Design review of the part built by this model. Coordinates are the model's own, in mm. A direction names the side the tool comes from. Give positions to 0.01 mm unless a question says otherwise; leave off trailing zeros. Loops run counter-clockwise (first coordinate to the right, second up) from the corner with the lowest first, then second, coordinate; pieces in that order, holes last.
from build123d import *

# Parameters (mm, degrees)
F0_R     = 2.38125
F0_W     = 0.79375
F0_H     = 1.5875
F1_DEPTH = 3.175
F2_DEPTH = 4.7625


with BuildPart() as f1:
    # F0 (on Top) → F1 (new body)
    with BuildSketch(Plane.XY):
        Polygon((3.96875, 3.96875), (-3.96875, 3.96875), (-3.96875, -3.96875), (-1.5875, -3.96875), (-0.79375, -3.96875), (0, -3.96875), (0.79375, -3.96875), (1.5875, -3.96875), (3.96875, -3.96875), align=None)
        Circle(F0_R, mode=Mode.SUBTRACT)
        Polygon((-0.79375, -3.96875), (-1.5875, -3.96875), (-1.5875, -5.55625), (0, -5.55625), (0, -3.96875), align=None)
        Polygon((1.5875, -5.55625), (1.5875, -3.96875), (0.79375, -3.96875), (0, -3.96875), (0, -5.55625), align=None)
        with BuildLine():
            Line((1.5875, -6.162621), (1.5875, -5.55625))
            Line((1.5875, -5.55625), (0, -5.55625))
            ThreePointArc((0, -5.55625), (0.849683, -5.713002), (1.5875, -6.162621))
        make_face()
        with BuildLine():
            Line((0, -5.55625), (-1.5875, -5.55625))
            Line((-1.5875, -5.55625), (-1.5875, -6.162621))
            ThreePointArc((-1.5875, -6.162621), (-0.849683, -5.713002), (0, -5.55625))
        make_face()
        with BuildLine():
            Line((0, -6.35), (0, -5.55625))
            ThreePointArc((0, -5.55625), (-0.849683, -5.713002), (-1.5875, -6.162621))
            ThreePointArc((-1.5875, -6.162621), (-2.173774, -6.965359), (-2.38125, -7.9375))
            Line((-2.38125, -7.9375), (-1.5875, -7.9375))
            ThreePointArc((-1.5875, -7.9375), (-1.122532, -6.814968), (0, -6.35))
        make_face()
        with Locations((-1.984375, -8.73125)):
            Rectangle(F0_W, F0_H)
        with BuildLine():
            ThreePointArc((1.5875, -6.162621), (0.849683, -5.713002), (0, -5.55625))
            Line((0, -5.55625), (0, -6.35))
            ThreePointArc((0, -6.35), (1.122532, -6.814968), (1.5875, -7.9375))
            Line((1.5875, -7.9375), (2.38125, -7.9375))
            ThreePointArc((2.38125, -7.9375), (2.173774, -6.965359), (1.5875, -6.162621))
        make_face()
        with Locations((1.984375, -8.73125)):
            Rectangle(F0_W, F0_H)
    extrude(amount=F1_DEPTH)

    # F0 (on Top) → F2 (join)
    with BuildSketch(Plane.XY):
        Circle(F0_R)
    extrude(amount=F2_DEPTH)


solid = f1.part
Q1. Insertion check: pin 1 (1.7 mm diameter, centred on y = -8.5, z = 1, fed in from -X); pin 2 (0.7 mm diameter, centred on x = 3, z = 1, fed in from -Y); pin 3 (0.8 mm diameter, centred on y = -9, z = 1.5, fed in from +X); pin 4 (1.2 mm diameter, centred on x = -2.5, z = 1, fed in from -Y) (3 decimals). Each pin has a flat end and moves straight along its axis. Give the tip position at first contact, or say it passes through.
Results:
pin 1: stops at x = -2.38
pin 2: stops at y = -3.97
pin 3: stops at x = 2.38
pin 4: stops at y = -9.525
Q2. Tool access review of faces 1 (the face through (-2.381, -9, 2)), 2 (the face through (2.381, -9, 2)), 3 (the face through (-1.588, -5, 2)): name each direction out of +Z, -Z, +X, -X, +Y, -Y from which nothing blocks a thin tool from reaching the whole face with its end or side.
Results:
face 1: +Z, -Z, -X, -Y
face 2: +Z, -Z, +X, -Y
face 3: +Z, -Z, -X
Q3. Take a section at A-A (x = -2). Give the boundary of the cut face in (y, z) (1 decimal).
Results:
outline: (-9.5, 0) - (-6.6, 0) - (-6.6, 3.2) - (-9.5, 3.2) - close; (-4, 0) - (4, 0) - (4, 3.2) - (1.3, 3.2) - (1.3, 4.8) - (-1.3, 4.8) - (-1.3, 3.2) - (-4, 3.2) - close
Q4. Take a section at D-D (y = 0). Give the boundary of the cut face in (x, z) (1 decimal), plus the area to 3 significant figures.
Results:
outline: (-4, 0) - (4, 0) - (4, 3.2) - (2.4, 3.2) - (2.4, 4.8) - (-2.4, 4.8) - (-2.4, 3.2) - (-4, 3.2) - close
area: 32.8 mm2
Q5. Wall thickness on line 1 (Z direction, x = 1.5, y = -6.25) (3 decimals); line 2 (X direction, y = -4, z = 0.65); line 3 (Y direction, x = -2.75, z = 2.25): over which ranges is each line inside the solid? List them lowest first.
Results:
line 1: z = 0 to 3.175
line 2: x = -1.59 to 1.59
line 3: y = -3.97 to 3.97
Q6. Take a section at B-B (y = -8.25). Give the boundary of the cut face in (x, z) (1 decimal).
Results:
outline: (-2.4, 0) - (-1.6, 0) - (-1.6, 3.2) - (-2.4, 3.2) - close; (1.6, 0) - (2.4, 0) - (2.4, 3.2) - (1.6, 3.2) - close
